Part model, mm, in its own coordinate system. Face numbers are marked on the shaded views. A direction names the side the tool comes from. Give positions to 0.01 mm unless a question says otherwise; leave off trailing zeros. Order: outer loops, then holes, each group sorted by start corner. A loop starts at its lowest first (then second) coordinate and runs counter-clockwise, first axis right, second up. Notation, with made-up numbers: (25.5, 25) -> (50.5, 25) arc R21 cw to (50.5, 57) -> close; hole circle Ø7 at (45, 85.25). An arc over 180 degrees is marked (long way). Write item = value, one per line. Start each with the question number.
(1) Two-plate mould, pull along Z, no slides. Class the marked faces 1, 2 and 3: pulls with the +Z half, pulls with the -Z half, needs draft (parallel to the pull), parting line crosses it, or undercut.
(2) Saw through at B-B, the plane z = -1.75. List the corners of the cut face in (x, y).
(3) Flat gauge pin, fed straight in: pin 1 (12 mm diameter, centred on x = 2, z = 6, fed in from -Y). Where does the tip first touch, or does it go through?
(4) Probe line 1 along Z through (x, y) = (-10, -198); line 2 along X through (y, z) = (-440, 9.85); line 3 along Y through (x, z) = (-15, 9.4). List the from-to ranges inside material, lowest first. Write a range as from..to.
(5) Saw through at A-A, the plane x = 9.5. List the corners of the cut face in (y, z), then the cut area to 3 significant figures.
(6) Saw through at C-C, the plane y = -89. List the corners of the cut face in (x, z), then the cut area to 3 significant figures.
(7) Which spindle directions (+Z, -Z, +X, -X, +Y, -Y) get a long thin tool onto all of the face, cutting with end or side? Do the marked faces 4 and 5. Say none if no direction does.
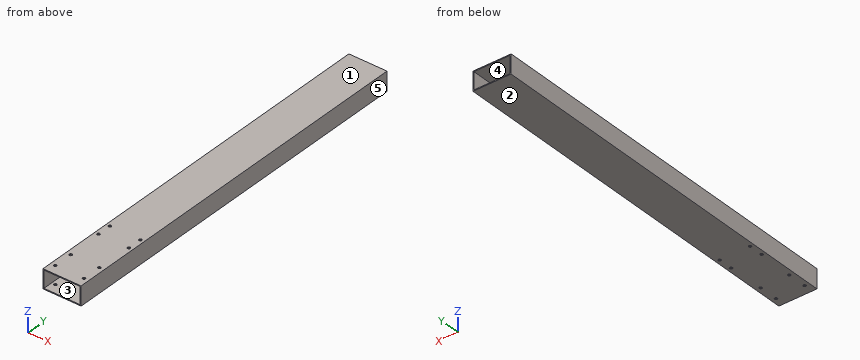
from build123d import *

# Parameters (mm, degrees)
SKETCH_12_W                   = 40
SKETCH_12_H                   = 20
SKETCH_12_W_2                 = 38
SKETCH_12_H_2                 = 18
F_20X40X1_LVGUAN20X40_1_DEPTH = 450
SKETCH_13_R                   = 1.5
CUT_EXTRUDE_1_DEPTH           = 51
SKETCH_14_W                   = 50.928856462
SKETCH_14_H                   = 27.036577468
CUT_EXTRUDE_2_DEPTH           = 50


with BuildPart() as part:
    # 草图12 → 20x40x1 LVGUAN20X40(1) (new body)
    with BuildSketch(Plane.XZ):
        Rectangle(SKETCH_12_W, SKETCH_12_H)
        Rectangle(SKETCH_12_W_2, SKETCH_12_H_2, mode=Mode.SUBTRACT)
    extrude(amount=F_20X40X1_LVGUAN20X40_1_DEPTH)

    # 草图13 → 切除-拉伸1 (cut)
    with BuildSketch(Plane.XY.offset(10)):
        with Locations((16, -382.5)):
            Circle(SKETCH_13_R)
        with Locations((16, -367.5)):
            Circle(SKETCH_13_R)
        with Locations((-16, -367.5)):
            Circle(SKETCH_13_R)
        with Locations((-16, -382.5)):
            Circle(SKETCH_13_R)
        with Locations((15, -420)):
            Circle(SKETCH_13_R)
        with Locations((-15, -420)):
            Circle(SKETCH_13_R)
        with Locations((-15, -440)):
            Circle(SKETCH_13_R)
        with Locations((15, -440)):
            Circle(SKETCH_13_R)
    extrude(amount=-CUT_EXTRUDE_1_DEPTH, mode=Mode.SUBTRACT)

    # 草图14 → 切除-拉伸2 (cut)
    with BuildSketch(Plane(origin=(0, 0, 0), x_dir=(1, 0, 0), z_dir=(0, 1, 0))):
        Rectangle(SKETCH_14_W, SKETCH_14_H)
    extrude(amount=-CUT_EXTRUDE_2_DEPTH, mode=Mode.SUBTRACT)


solid = part.part
Results list:
q1.face_1 = pulls with the +Z half
q1.face_2 = pulls with the -Z half
q1.face_3 = undercut
q2.outline = (-20, -450) -> (-19, -450) -> (-19, -50) -> (-20, -50) -> close; (19, -450) -> (20, -450) -> (20, -50) -> (19, -50) -> close
q3.pin_1 = -450
q4.line_1 = -10..-9, 9..10
q4.line_2 = -20..-16.5, -13.5..13.5, 16.5..20
q4.line_3 = -450..-441.5, -438.5..-421.5, -418.5..-383.62, -381.38..-368.62, -366.38..-50
q5.outline = (-450, -10) -> (-50, -10) -> (-50, -9) -> (-450, -9) -> close; (-450, 9) -> (-50, 9) -> (-50, 10) -> (-450, 10) -> close
q5.area = 800 mm^2
q6.outline = (-20, -10) -> (20, -10) -> (20, 10) -> (-20, 10) -> close; hole (-19, -9) -> (19, -9) -> (19, 9) -> (-19, 9) -> close
q6.area = 116 mm^2
q7.face_4 = +Y, -Y
q7.face_5 = +Z, -Z, +X, +Y, -Y
